from build123d import *

# Parameters (mm, degrees)
F1_DEPTH  = 19.05
F2_R      = 25.4
F4_DEPTH  = 527.051
F6_W      = 101.854
F6_H      = 19.2786
F7_DEPTH  = 231.9562403073
F9_W      = 202.692
F9_H      = 19.2786
F10_DEPTH = 210.9250403073


with BuildPart() as f1:
    # F0 (on Top) → F1 (new body)
    with BuildSketch(Plane.XY):
        Polygon((0, 101.6), (0, 0), (508, 0), (508, 101.6), (527.05, 101.6), (527.05, 152.4), (527.05, 203.2), (508, 203.2), (508, 304.8), (527.05, 304.8), (527.05, 355.6), (527.05, 406.4), (508, 406.4), (508, 508), (254, 508), (0, 508), (0, 406.4), (-19.05, 406.4), (-19.05, 355.6), (-19.05, 304.8), (0, 304.8), (0, 203.2), (-19.05, 203.2), (-19.05, 152.4), (-19.05, 101.6), align=None)
    extrude(amount=F1_DEPTH)

    # F2
    f2_edges = [f1.edges().sort_by_distance(p)[0] for p in [
        (0, 508, 9.525),
        (508, 508, 9.525),
    ]]
    fillet(f2_edges, radius=F2_R)

    # F3 (on face) → F4 (cut, through all)
    with BuildSketch(Plane(origin=(0, 0, 0), x_dir=(0, -1, 0), z_dir=(-1, 0, 0))):
        Polygon((0, 0), (0, 19.05), (-8.8831608879, 0), align=None)
    extrude(amount=-F4_DEPTH, mode=Mode.SUBTRACT)

    # F6 (on face) → F7 (cut, through all)
    with BuildSketch(Plane(origin=(0, -7.2965733207, 15.6475519823), x_dir=(1, 0, 0), z_dir=(0, 0.4226182617, -0.906307787))):
        with Locations((101.727, -17.6901778862)):
            Rectangle(F6_W, F6_H)
        with Locations((406.273, -17.6901778862)):
            Rectangle(F6_W, F6_H)
    extrude(amount=F7_DEPTH, mode=Mode.SUBTRACT)

    # F9 (on face) → F10 (cut, through all)
    with BuildSketch(Plane(origin=(0, 1.5915958656, -3.4131883485), x_dir=(1, 0, 0), z_dir=(0, 0.4226182617, -0.906307787))):
        with Locations((254, -17.6901778862)):
            Rectangle(F9_W, F9_H)
    extrude(amount=F10_DEPTH, mode=Mode.SUBTRACT)


solid = f1.part
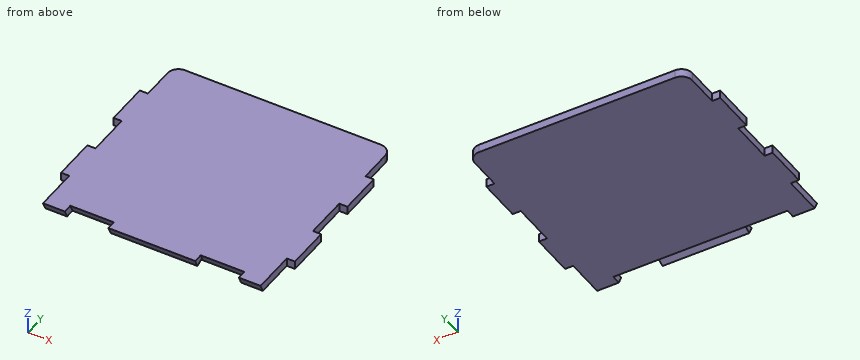
Can you work these out from the model? Positions are in its coordinate system, mm. Coordinates: 2 decimals unless noted, no trailing zeros. Order: outer loops, then holes, each group sorted by start corner. A loop starts at its lowest first (then second) coordinate and runs counter-clockwise, first axis right, second up. Notation, with made-up numbers: M 46,82.5 L 53,82.5 A24 cw 53,119.5 Z; hole C 33.25,11 d4. An arc over 180 degrees is marked long. Answer as CSV lines item,"result".
(1) Suppose I cut it at C-C on y = 90.5. Please give me the cut outline in (x, z), plus the area to 3 significant figures.
Geometry check:
outline,"M 0,0 L 508,0 L 508,19.05 L 0,19.05 Z"
area,"9,680 mm^2"
(2) I'm going to push flat-ended pins straight in: pin 1 (5.5 mm diameter, centred on y = 276, z = 7.5, fed in from -X); pin 2 (10 mm diameter, centred on x = 63, z = 3.5, fed in from -Y); pin 3 (5.5 mm diameter, centred on x = -8, z = 5.5, fed in from +Y). Where does each tip first touch, or does it pass through?
Geometry check:
pin 1,"x = 0"
pin 2,"y = 26.19"
pin 3,"y = 406.4"
(3) Please list where these lines run through material, in increasing order: L1, parallel to X at y = 278, z = 15.25; L2, parallel to Y at x = 482.5, z = 17.5; L3, parallel to Y at x = 191.5, z = 8.5.
Geometry check:
L1,"0 to 508"
L2,"0.72 to 508"
L3,"4.92 to 508"
